Geometry check sheet. Reference: the model listing, model coordinates, mm. A direction names the side the tool comes from. Give positions to 0.01 mm unless a question says otherwise; leave off trailing zeros. Loops run counter-clockwise (first coordinate to the right, second up) from the corner with the lowest first, then second, coordinate; pieces in that order, holes last. Notation, with made-up numbers: (-20.5, -1.75) - (19.5, -1.75) arc R25 ccw to (19.5, 32.25) - close; hole circle Ø10 at (80, 86). An arc over 180 degrees is marked (long way). Write item = value, one per line. Start each with the question number.
from build123d import *

# Parameters (mm, degrees)
TUBE004_R         = 3
TUBE004_R_2       = 1.5
TUBE004_DEPTH     = 10.35
TUBE002_R         = 3
TUBE002_R_2       = 1.5
TUBE002_DEPTH     = 10.35
TUBE001_R         = 3
TUBE001_R_2       = 1.5
TUBE001_DEPTH     = 10.35
TUBE_R            = 3
TUBE_R_2          = 1.5
TUBE_DEPTH        = 10.35
CYLINDER007_R     = 1.5
CYLINDER007_DEPTH = 2
CYLINDER006_R     = 1.5
CYLINDER006_DEPTH = 2
CYLINDER005_R     = 1.5
CYLINDER005_DEPTH = 2
CYLINDER004_R     = 1.5
CYLINDER004_DEPTH = 2
BOX012_W          = 1
BOX012_H          = 1
BOX012_DEPTH      = 1
BOX011_W          = 13
BOX011_H          = 24.2
BOX011_DEPTH      = 10
BOX010_W          = 10
BOX010_H          = 24
BOX010_DEPTH      = 10
BOX009_W          = 5
BOX009_H          = 12
BOX009_DEPTH      = 10
BOX008_W          = 8
BOX008_H          = 48
BOX008_DEPTH      = 10
BOX007_W          = 109
BOX007_H          = 67
BOX007_DEPTH      = 1
BOX006_W          = 111
BOX006_H          = 69
BOX006_DEPTH      = 1
BOX005_W          = 109
BOX005_H          = 67
BOX005_DEPTH      = 6
BOX004_W          = 113
BOX004_H          = 71
BOX004_DEPTH      = 8


with BuildPart() as obj1:
    # Tube004 → Tube004 (new body)
    with BuildSketch(Plane(origin=(103.69, -64.33, -0.35), x_dir=(1, 0, 0), z_dir=(0, 0, 1))):
        Circle(TUBE004_R)
        Circle(TUBE004_R_2, mode=Mode.SUBTRACT)
    extrude(amount=TUBE004_DEPTH)


with BuildPart() as obj2:
    # Tube002 → Tube002 (new body)
    with BuildSketch(Plane(origin=(93.54, -8.44, -0.35), x_dir=(1, 0, 0), z_dir=(0, 0, 1))):
        Circle(TUBE002_R)
        Circle(TUBE002_R_2, mode=Mode.SUBTRACT)
    extrude(amount=TUBE002_DEPTH)


with BuildPart() as obj3:
    # Tube001 → Tube001 (new body)
    with BuildSketch(Plane(origin=(9.71, -64.33, -0.35), x_dir=(1, 0, 0), z_dir=(0, 0, 1))):
        Circle(TUBE001_R)
        Circle(TUBE001_R_2, mode=Mode.SUBTRACT)
    extrude(amount=TUBE001_DEPTH)


with BuildPart() as pusher_lo:
    # Tube → Tube (new body)
    with BuildSketch(Plane(origin=(9.71, -8.44, -0.35), x_dir=(1, 0, 0), z_dir=(0, 0, 1))):
        Circle(TUBE_R)
        Circle(TUBE_R_2, mode=Mode.SUBTRACT)
    extrude(amount=TUBE_DEPTH)


with BuildPart() as obj4:
    # Cylinder007 → Cylinder007 (new body)
    with BuildSketch(Plane(origin=(103.69, -64.33, 10), x_dir=(1, 0, 0), z_dir=(0, 0, 1))):
        Circle(CYLINDER007_R)
    extrude(amount=CYLINDER007_DEPTH)


with BuildPart() as obj5:
    # Cylinder006 → Cylinder006 (new body)
    with BuildSketch(Plane(origin=(93.54, -8.44, 10), x_dir=(1, 0, 0), z_dir=(0, 0, 1))):
        Circle(CYLINDER006_R)
    extrude(amount=CYLINDER006_DEPTH)


with BuildPart() as obj6:
    # Cylinder005 → Cylinder005 (new body)
    with BuildSketch(Plane(origin=(9.71, -64.33, 10), x_dir=(1, 0, 0), z_dir=(0, 0, 1))):
        Circle(CYLINDER005_R)
    extrude(amount=CYLINDER005_DEPTH)


with BuildPart() as hole_lo:
    # Cylinder004 → Cylinder004 (new body)
    with BuildSketch(Plane(origin=(9.71, -8.44, 10), x_dir=(1, 0, 0), z_dir=(0, 0, 1))):
        Circle(CYLINDER004_R)
    extrude(amount=CYLINDER004_DEPTH)


with BuildPart() as supply_cut:
    # Box012 → Box012 (new body)
    with BuildSketch(Plane(origin=(86, -70, 9), x_dir=(1, 0, 0), z_dir=(0, 0, 1))):
        with Locations((0.5, 0.5)):
            Rectangle(BOX012_W, BOX012_H)
    extrude(amount=BOX012_DEPTH)


with BuildPart() as phoenix_cut:
    # Box011 → Box011 (new body)
    with BuildSketch(Plane(origin=(95.5, -34.6, 3), x_dir=(1, 0, 0), z_dir=(0, 0, 1))):
        with Locations((6.5, 12.1)):
            Rectangle(BOX011_W, BOX011_H)
    extrude(amount=BOX011_DEPTH)


with BuildPart() as obj7:
    # Box010 → Box010 (new body)
    with BuildSketch(Plane(origin=(98, -60, 3), x_dir=(1, 0, 0), z_dir=(0, 0, 1))):
        with Locations((5, 12)):
            Rectangle(BOX010_W, BOX010_H)
    extrude(amount=BOX010_DEPTH)


with BuildPart() as box009:
    # Box009 → Box009 (new body)
    with BuildSketch(Plane(origin=(12, -43, 6), x_dir=(1, 0, 0), z_dir=(0, 0, 1))):
        with Locations((2.5, 6)):
            Rectangle(BOX009_W, BOX009_H)
    extrude(amount=BOX009_DEPTH)


with BuildPart() as box008:
    # Box008 → Box008 (new body)
    with BuildSketch(Plane(origin=(6, -61, 6), x_dir=(1, 0, 0), z_dir=(0, 0, 1))):
        with Locations((4, 24)):
            Rectangle(BOX008_W, BOX008_H)
    extrude(amount=BOX008_DEPTH)


with BuildPart() as casebottomlip_in001:
    # Box007 → Box007 (new body)
    with BuildSketch(Plane(origin=(2, -70, -13), x_dir=(1, 0, 0), z_dir=(0, 0, 1))):
        with Locations((54.5, 33.5)):
            Rectangle(BOX007_W, BOX007_H)
    extrude(amount=BOX007_DEPTH)


with BuildPart() as casetoplip:
    # Box006 → Box006 (new body)
    with BuildSketch(Plane(origin=(1, -71, -13), x_dir=(1, 0, 0), z_dir=(0, 0, 1))):
        with Locations((55.5, 34.5)):
            Rectangle(BOX006_W, BOX006_H)
    extrude(amount=BOX006_DEPTH)

    # Cut003: cut CaseBottomLip_In001
    add(casebottomlip_in001.part, mode=Mode.SUBTRACT)


with BuildPart() as casetopbed_in:
    # Box005 → Box005 (new body)
    with BuildSketch(Plane(origin=(2, -70, -12), x_dir=(1, 0, 0), z_dir=(0, 0, 1))):
        with Locations((54.5, 33.5)):
            Rectangle(BOX005_W, BOX005_H)
    extrude(amount=BOX005_DEPTH)


with BuildPart() as casetop:
    # Box004 → Box004 (new body)
    with BuildSketch(Plane(origin=(0, -72, -12), x_dir=(1, 0, 0), z_dir=(0, 0, 1))):
        with Locations((56.5, 35.5)):
            Rectangle(BOX004_W, BOX004_H)
    extrude(amount=BOX004_DEPTH)

    # Cut002: cut CaseTopBed_In
    add(casetopbed_in.part, mode=Mode.SUBTRACT)

    # Fusion001: union CaseTopLip
    add(casetoplip.part)


with BuildPart() as casetop_1:
    # Fusion001 placement: moved
    add(casetop.part.moved(Location((0, 0, 16))))

    # Cut004: cut Box008
    add(box008.part, mode=Mode.SUBTRACT)

    # Cut005: cut Box009
    add(box009.part, mode=Mode.SUBTRACT)

    # Cut006: cut obj7
    add(obj7.part, mode=Mode.SUBTRACT)

    # Cut007: cut Phoenix_Cut
    add(phoenix_cut.part, mode=Mode.SUBTRACT)

    # Cut008: cut Supply_Cut
    add(supply_cut.part, mode=Mode.SUBTRACT)

    # Cut013: cut Hole_LO
    add(hole_lo.part, mode=Mode.SUBTRACT)

    # Cut014: cut obj6
    add(obj6.part, mode=Mode.SUBTRACT)

    # Cut015: cut obj5
    add(obj5.part, mode=Mode.SUBTRACT)

    # Cut016: cut obj4
    add(obj4.part, mode=Mode.SUBTRACT)

    # Fusion006: union Pusher_LO
    add(pusher_lo.part)

    # Fusion007: union obj3
    add(obj3.part)

    # Fusion008: union obj2
    add(obj2.part)

    # Fusion009: union obj1
    add(obj1.part)


with BuildPart() as casetop_2:
    # Fusion009 placement: moved
    add(casetop_1.part.moved(Location((0, 0, 13))))


solid = casetop_2.part
1) Cross-section at D-D on x = 93.54. Enter the section's corners in (y, z), and give its area (3 significant figures).
2) Gauge pin test, flat ends, axial feed: P1, Ø0.5, axis at y = -40.5, z = 16.5, coming from the +X side; P2, Ø20.5, axis at x = 32, y = -47, coming from the -Z side; P3, Ø0.8, axis at x = 62.5, z = 16.5, coming from the +Y side. Record the tip position at first contact, or that the pin passes through.
3) Tool access check on faces 1 (the face through (90.543, -8.308, 17.753)), 2 (the face through (94.23, -9.77, 18.74)). Record the directions out of +Z, -Z, +X, -X, +Y, -Y that give a thin tool (end or side, any length) a straight path to the whole face; none if there is none.
4) Release check for a two-part mould opening along X. For faces 3 (the face through (56, -36, 25)), 4 (the face through (9.06, -67.26, 17.75)), 5 (the face through (113, -37, 21)) record: pulls with the +X half, pulls with the -X half, needs draft (parallel to the pull), parting line crosses it, or undercut.
5) Material ranges on line 1 along X through (y, z) = (-41, 24.25); line 2 along X through (y, z) = (-49.5, 24.25); line 3 along Y through (x, z) = (93.54, 21.5), recorded low to high.
6) Cross-section at C-C on y = -64.33. Enter the section's corners in (x, z), and give its area (3 significant figures).
7) Cross-section at A-A on z = 18.75. Give the number of separate pieces and of enclosed holes in the cut face, and give its area (3 significant figures).
Checked values:
q1.outline = (-72, 17) - (-71, 17) - (-71, 16) - (-70, 16) - (-70, 23) - (-11.44, 23) - (-11.44, 12.65) - (-9.94, 12.65) - (-9.94, 25) - (-72, 25) - close; (-6.94, 12.65) - (-5.44, 12.65) - (-5.44, 23) - (-3, 23) - (-3, 16) - (-2, 16) - (-2, 17) - (-1, 17) - (-1, 25) - (-6.94, 25) - close
q1.area = 193 mm²
q2.P1 = 112
q2.P2 = 23
q2.P3 = -2
q3.face_1 = -Z
q3.face_2 = +Z, -Z
q4.face_3 = needs draft
q4.face_4 = undercut
q4.face_5 = pulls with the +X half
q5.line_1 = 0 to 6, 17 to 98, 108 to 113
q5.line_2 = 0 to 6, 14 to 98, 108 to 113
q5.line_3 = -72 to -70, -11.44 to -9.94, -6.94 to -5.44, -3 to -1
q6.outline = (0, 17) - (1, 17) - (1, 16) - (2, 16) - (2, 23) - (6.71, 23) - (6.71, 12.65) - (8.21, 12.65) - (8.21, 25) - (0, 25) - close; (11.21, 12.65) - (12.71, 12.65) - (12.71, 23) - (100.69, 23) - (100.69, 12.65) - (102.19, 12.65) - (102.19, 25) - (11.21, 25) - close; (105.19, 12.65) - (106.69, 12.65) - (106.69, 23) - (111, 23) - (111, 16) - (112, 16) - (112, 17) - (113, 17) - (113, 25) - (105.19, 25) - close
q6.area = 302 mm²
q7.separate_pieces = 5
q7.enclosed_holes = 5
q7.area = 805 mm²
